```python
from build123d import *

# Parameters (mm, degrees)
SKETCH008_R         = 0.5
PAD004_DEPTH        = 2.6
SKETCH009_R         = 3
SKETCH009_R_2       = 0.5
PAD005_DEPTH        = 4
HOLE004_D           = 2.8
HOLE004_CSINK_D     = 3.8
HOLE004_CSINK_ANGLE = 90
HOLE005_D           = 2.3
HOLE005_CSINK_D     = 3.3
HOLE005_CSINK_ANGLE = 90
HOLE006_D           = 3.2
HOLE006_CBORE_D     = 6
HOLE006_CBORE_DEPTH = 1.7


with BuildPart() as part:
    # Sketch008 → Pad004 (new body)
    with BuildSketch(Plane.XY):
        with BuildLine():
            ThreePointArc((-30.94, 13.16), (-33.06132, 12.28132), (-33.94, 10.16))
            Line((-33.94, -10.16), (-33.94, 10.16))
            ThreePointArc((-33.94, -10.16), (-33.06132, -12.28132), (-30.94, -13.16))
            Line((30.94, -13.16), (-30.94, -13.16))
            ThreePointArc((30.94, -13.16), (33.06132, -12.28132), (33.94, -10.16))
            Line((33.94, 10.16), (33.94, -10.16))
            ThreePointArc((33.94, 10.16), (33.06132, 12.28132), (30.94, 13.16))
            Line((-30.94, 13.16), (30.94, 13.16))
        make_face()
        with Locations((-30.94, 10.16)):
            Circle(SKETCH008_R, mode=Mode.SUBTRACT)
        with Locations((-10.62, 10.16)):
            Circle(SKETCH008_R, mode=Mode.SUBTRACT)
        with Locations((-2.54, 10.16)):
            Circle(SKETCH008_R, mode=Mode.SUBTRACT)
        with Locations((10.16, 10.16)):
            Circle(SKETCH008_R, mode=Mode.SUBTRACT)
        with Locations((18.24, 10.16)):
            Circle(SKETCH008_R, mode=Mode.SUBTRACT)
        with Locations((30.94, 10.16)):
            Circle(SKETCH008_R, mode=Mode.SUBTRACT)
        with Locations((-30.94, -10.16)):
            Circle(SKETCH008_R, mode=Mode.SUBTRACT)
        with Locations((-10.62, -10.16)):
            Circle(SKETCH008_R, mode=Mode.SUBTRACT)
        with Locations((-2.54, -10.16)):
            Circle(SKETCH008_R, mode=Mode.SUBTRACT)
        with Locations((10.16, -10.16)):
            Circle(SKETCH008_R, mode=Mode.SUBTRACT)
        with Locations((18.24, -10.16)):
            Circle(SKETCH008_R, mode=Mode.SUBTRACT)
        with Locations((30.94, -10.16)):
            Circle(SKETCH008_R, mode=Mode.SUBTRACT)
    extrude(amount=PAD004_DEPTH)

    # Sketch009 (on Face22 of Pad004) → Pad005 (join)
    with BuildSketch(Plane.XY.offset(2.6)):
        with Locations((-30.94, 10.16)):
            Circle(SKETCH009_R)
        with Locations((-30.94, 10.16)):
            Circle(SKETCH009_R_2, mode=Mode.SUBTRACT)
        with Locations((30.94, 10.16)):
            Circle(SKETCH009_R)
        with Locations((30.94, 10.16)):
            Circle(SKETCH009_R_2, mode=Mode.SUBTRACT)
        with BuildLine():
            ThreePointArc((-10.62, 13.16), (-13.62, 10.16), (-10.62, 7.16))
            Line((-10.62, 7.16), (-2.54, 7.16))
            ThreePointArc((-2.54, 7.16), (0.46, 10.16), (-2.54, 13.16))
            Line((-2.54, 13.16), (-10.62, 13.16))
        make_face()
        with Locations((-10.62, 10.16)):
            Circle(SKETCH009_R_2, mode=Mode.SUBTRACT)
        with Locations((-2.54, 10.16)):
            Circle(SKETCH009_R_2, mode=Mode.SUBTRACT)
        with BuildLine():
            ThreePointArc((10.16, 13.16), (7.16, 10.16), (10.16, 7.16))
            Line((10.16, 7.16), (18.24, 7.16))
            ThreePointArc((18.24, 7.16), (21.24, 10.16), (18.24, 13.16))
            Line((18.24, 13.16), (10.16, 13.16))
        make_face()
        with Locations((10.16, 10.16)):
            Circle(SKETCH009_R_2, mode=Mode.SUBTRACT)
        with Locations((18.24, 10.16)):
            Circle(SKETCH009_R_2, mode=Mode.SUBTRACT)
    pad005 = extrude(amount=PAD005_DEPTH)

    # Hole004 (through all)
    with Locations(Plane.XY.offset(6.6)):
        with Locations((-30.94, 10.16), (-10.62, 10.16)):
            hole004 = CounterSinkHole(HOLE004_D / 2, HOLE004_CSINK_D / 2, counter_sink_angle=HOLE004_CSINK_ANGLE)

    # Hole005 (through all)
    with Locations(Plane.XY.offset(6.6)):
        with Locations((-2.54, 10.16), (10.16, 10.16), (18.24, 10.16), (30.94, 10.16)):
            hole005 = CounterSinkHole(HOLE005_D / 2, HOLE005_CSINK_D / 2, counter_sink_angle=HOLE005_CSINK_ANGLE)

    # Mirrored004: Pad005, Hole004, Hole005 across Sketch009 H_Axis
    add(pad005.mirror(Plane(origin=(0, 0, 2.6), x_dir=(0, 0, 1), z_dir=(0, 1, 0))))
    add(hole004.mirror(Plane(origin=(0, 0, 2.6), x_dir=(0, 0, 1), z_dir=(0, 1, 0))), mode=Mode.SUBTRACT)
    add(hole005.mirror(Plane(origin=(0, 0, 2.6), x_dir=(0, 0, 1), z_dir=(0, 1, 0))), mode=Mode.SUBTRACT)

    # Hole006 (through all)
    with Locations(Plane.XY.offset(2.6)):
        with Locations((-25.5, 0), (25.5, 0)):
            CounterBoreHole(HOLE006_D / 2, HOLE006_CBORE_D / 2, HOLE006_CBORE_DEPTH)


solid = part.part
```
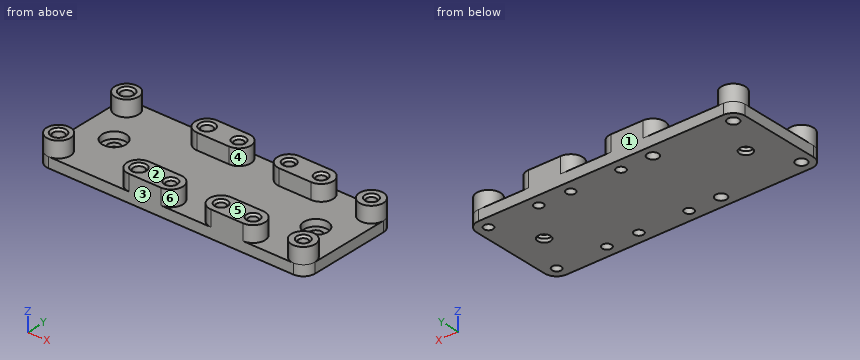
Source: CAD feature listing. Evaluate the final solid. Frame: model axes, mm. Face numbers are marked on the shaded views. A direction names the side the tool comes from. Round coordinates to 2 decimals unless told otherwise and drop trailing zeros. Loops run counter-clockwise (first coordinate to the right, second up) from the corner with the lowest first, then second, coordinate; pieces in that order, holes last. Notation, with made-up numbers: M 22.25,-38 L 56.25,-38 A8 cw 56.25,-24 Z; hole C 3,-4.75 d1. An arc over 180 degrees is marked long. Use a Markdown table: item, result. Add a question column.
1. Section query C-C on y = 0. Return the cut outline in (x, z), then the cut area to 3 significant figures.
2. Line query: line 1 (Y direction, x = -30.94, z = 5); line 2 (Y direction, x = 30.94, z = 1.5); line 3 (Y direction, x = 30.94, z = 3). Output: solid intervals per line, ascending.
3. Section query A-A on z = 4.75. Give the number of separate pieces and of enclosed holes in the cut face, then the cut area to 3 significant figures.
4. Section query D-D on x = -26. Return the cut outline in (y, z), then the cut area to 3 significant figures.
5. Section query B-B on x = 25.5. Return the cut outline in (y, z).
6. Mould query, pull axis Y, two halves, no side actions, for the marked faces 1, 2, 3 and 4. Classes: pulls with the +Y half, pulls with the -Y half, needs draft (parallel to the pull), parting line crosses it, or undercut.
7. Reachability of the marked faces 5 and 6 from +Z, -Z, +X, -X, +Y, -Y: full face, straight path, thin tool, end or side. Return the list, or none.
8. Contact query for flat-ended pins moving along their axis: P1, Ø3, axis at y = -6, z = 5, coming from the +X side; P2, Ø3, axis at y = 2.5, z = 4.5, coming from the -X side; P3, Ø2.5, axis at x = -2.54, y = -10.16, coming from the +Z side; P4, Ø5, axis at x = -25.5, y = 0, coming from the +Z side. Output: stop coordinate, or through.
Reported:
| question | item | result |
|---|---|---|
| 1 | outline | M -33.94,0 L -27.1,0 L -27.1,0.9 L -28.5,0.9 L -28.5,2.6 L -33.94,2.6 Z; M -23.9,0 L 23.9,0 L 23.9,0.9 L 22.5,0.9 L 22.5,2.6 L -22.5,2.6 L -22.5,0.9 L -23.9,0.9 Z; M 27.1,0 L 33.94,0 L 33.94,2.6 L 28.5,2.6 L 28.5,0.9 L 27.1,0.9 Z |
| 1 | area | 150 mm² |
| 2 | line 1 | y = -13.16 to -11.56, -8.76 to -7.16, 7.16 to 8.76, 11.56 to 13.16 |
| 2 | line 2 | y = -13.16 to -11.31, -9.01 to 9.01, 11.31 to 13.16 |
| 2 | line 3 | y = -13.16 to -11.31, -9.01 to -7.16, 7.16 to 9.01, 11.31 to 13.16 |
| 3 | separate pieces | 8 |
| 3 | enclosed holes | 12 |
| 3 | area | 362 mm² |
| 4 | outline | M -13.16,0 L -1.52,0 L -1.52,0.9 L -2.96,0.9 L -2.96,2.6 L -13.16,2.6 Z; M 1.52,0 L 13.16,0 L 13.16,2.6 L 2.96,2.6 L 2.96,0.9 L 1.52,0.9 Z |
| 4 | area | 55.6 mm² |
| 5 | outline | M -13.16,0 L -1.6,0 L -1.6,0.9 L -3,0.9 L -3,2.6 L -13.16,2.6 Z; M 1.6,0 L 13.16,0 L 13.16,2.6 L 3,2.6 L 3,0.9 L 1.6,0.9 Z |
| 6 | face 1 | pulls with the +Y half |
| 6 | face 2 | needs draft |
| 6 | face 3 | pulls with the -Y half |
| 6 | face 4 | undercut |
| 7 | face 5 | +Z, +X, -X, +Y, -Y |
| 7 | face 6 | +Z |
| 8 | P1 | stops at x = 32.33 |
| 8 | P2 | passes through |
| 8 | P3 | stops at z = 6.2 |
| 8 | P4 | stops at z = 0.9 |
